Autodesk Inventor part; units mm, degrees
ref_plane "Arbeitsebene1" through (0, 0, 8) normal (0, 0, 1) x (1, 0, 0)
ref_plane "YZ Plane" through (0, 0, 0) normal (1, 0, 0) x (0, 1, 0)
ref_plane "XZ Plane" through (0, 0, 0) normal (0, 1, 0) x (-1, 0, 0)
sketch "Skizze1" plane through (0, 0, 0) normal (0, 0, 1) x (1, 0, 0)
  line L0 (-31.2, 0) -> (-31.2, 8)
  line L1 (-31.2, 8) -> (-27.8, 8)
  line L2 (-27.8, 8) -> (-27.8, 7.15)
  line L3 (-27.8, 7.15) -> (-26.5, 7.15)
  line L4 (-26.5, 7.15) -> (-26.5, 8)
  line L5 (-26.5, 8) -> (23.2, 8)
  line L6 (23.2, 8) -> (23.2, 14)
  line L7 (23.2, 14) -> (31.2, 14)
  line L8 (31.2, 14) -> (31.2, 0)
  line L9 (-43.68, 0) -> (43.68, 0)
  line L10 (0, -2.8) -> (0, 16.8)
  line L11 (-31.2, 0) -> (31.2, 0)
  point P0 (0, 0)
  dimension "d0" = 49.7
  dimension "d1" = 8
  dimension "d2" = 6
  dimension "d3" = 1.3
  dimension "d4" = 0.85
  dimension "d5" = 3.4
  dimension "d6" = 8
revolve "Umdrehung1" add sketch "Skizze1" angle 360 about axis through (-10, 0, 0) along (1, 0, 0)
chamfer "Fase1" distance 2 angle 45 1 edges at (-31.2, -8, 0)
chamfer "Fase2" distance 1 angle 45 1 edges at (31.2, -14, 0)
chamfer "Fase3" distance 1 angle 45 1 edges at (23.2, -14, 0)
sketch "Skizze4" plane through (-31.2, 0, 0) normal (-1, 0, 0) x (0, 0, 1)
  point P0 (0, 0)
  point P1 (0, 0)
hole "Bohrung2" at (-31.2, 0, 0) direction (1, 0, 0) diameter 5 depth 35 tip angle 118
ref_plane "Arbeitsebene1" through (0, 0, 8) normal (0, 0, 1) x (1, 0, 0)
sketch "Skizze5" plane through (0, 0, 8) normal (0, 0, 1) x (1, 0, 0)
  line L0 (-2.4, 0) -> (0.4, 0)
  point P0 (0, 0)
  point P1 (-2, 0)
  dimension "d46" = 2
hole "Bohrung3" at (-2, 0, 8) direction (0, 0, -1) diameter 4 end through all
thread "Gewinde1"
properties part number "KON_Nietmaschine_Bolzen" material "Stahl"
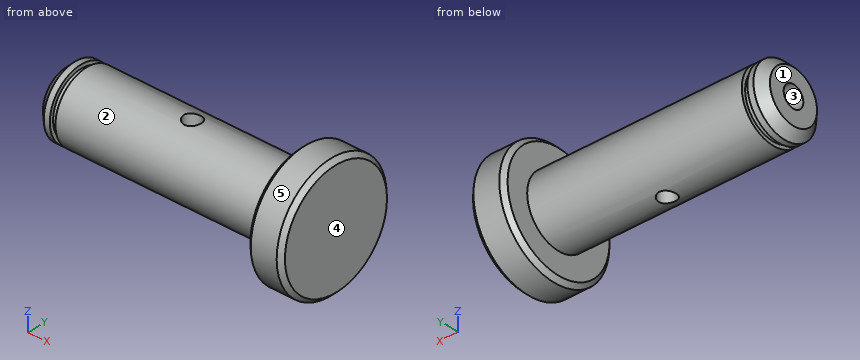
Model file for the job. Use its own axes, mm. Face numbers are marked on the shaded views. A direction names the side the tool comes from. Coordinates: 2 decimals unless noted, no trailing zeros. Order: outer loops, then holes, each group sorted by start corner. A loop starts at its lowest first (then second) coordinate and runs counter-clockwise, first axis right, second up. Notation, with made-up numbers: (-33.5, 42) - (-3.5, 42) arc R30 cw to (-3.5, 78) - close; hole circle Ø4 at (-3.5, 61.5). An arc over 180 degrees is marked (long way). Return JSON: item names as keys, results as strings. Group by question number.
1) Mould opens along Y. For the marked faces 3, 4 and 5 say: released by +Y, released by -Y, zero draft, split by the parting line, or undercut.
2) Tool access for the marked faces 1 and 2: list every direction of +Z, -Z, +X, -X, +Y, -Y with a clear straight run to the whole face (end or side of a thin tool).
3) Probe line 1 (X direction, y = 0, z = -6); line 2 (Y direction, x = 1.5, z = -1.75); line 3 (X direction, y = 9.5, z = 5). List the from-to ranges inside material, lowest first. Write a range as from..to.
4) Saw through at B-B, the plane x = 26.5. Write the cut outline in (y, z).
5) Flat gauge pins, fed straight in: P1, Ø1, axis at x = 23, z = 1.5, coming from the +Y side; P2, Ø1, axis at x = -7.5, z = 0.5, coming from the +Y side; P3, Ø6.5, axis at x = -2, y = 0, coming from the +Z side. Where does each tip first touch, or does it go through?
6) Saw through at A-A, the plane x = -1. Write the cut outline in (y, z).
Values found:
{
 "1": {"face 3": "undercut", "face 4": "zero draft", "face 5": "split by the parting line"},
 "2": {"face 1": "+Z, -Z, -X, +Y, -Y", "face 2": "-X"},
 "3": {"line 1": "x = -31.2..-4, 0..31.2", "line 2": "y = -7.81..-1.79, 1.79..7.81", "line 3": "x = 23.2..31.2"},
 "4": {"outline": "circle Ø28 at (0, 0)"},
 "5": {"P1": "stops at y = 13.22", "P2": "stops at y = 8", "P3": "stops at z = 8"},
 "6": {"outline": "(-1.73, -7.81) - (-1.73, -1.8) arc R2.5 cw to (-1.73, 1.8) - (-1.73, 7.81) arc R8 ccw to start; (1.73, -7.81) arc R8 ccw to (1.73, 7.81) - (1.73, 1.8) arc R2.5 cw to (1.73, -1.8) - close"}
}
